from build123d import *

# Parameters (mm, degrees)
SKETCH1_R                = 1.6
SKETCH1_R_2              = 15.5
BOSS_EXTRUDE1_DEPTH      = 3
SKETCH2_W                = 12.85
SKETCH2_H                = 3
BOSS_EXTRUDE2_DEPTH      = 25
SKETCH3_R                = 1.6
CUT_EXTRUDE1_DEPTH       = 4
BOSS_EXTRUDE3_DEPTH      = 3
CHAMFER1_SIZE            = 2
FILLET1_R                = 3
FILLET2_R                = 3
CHAMFER1_OF_MIRROR1_SIZE = 2
FILLET1_OF_MIRROR1_R     = 3


with BuildPart() as part:
    # Sketch1 → Boss-Extrude1 (new body)
    with BuildSketch(Plane(origin=(0, 0, 0), x_dir=(1, 0, 0), z_dir=(0, 1, 0))):
        Polygon((46.15, 13.849265428), (-46.15, 13.849265428), (-59, -25.450734572), (-59, -28.450734572), (59, -28.450734572), (59, -25.450734572), align=None)
        with Locations((-40.5, 8.199265428)):
            Circle(SKETCH1_R, mode=Mode.SUBTRACT)
        with Locations((-9.5, 8.199265428)):
            Circle(SKETCH1_R, mode=Mode.SUBTRACT)
        with Locations((-40.5, -22.800734572)):
            Circle(SKETCH1_R, mode=Mode.SUBTRACT)
        with Locations((-9.5, -22.800734572)):
            Circle(SKETCH1_R, mode=Mode.SUBTRACT)
        with Locations((-25, -7.300734572)):
            Circle(SKETCH1_R_2, mode=Mode.SUBTRACT)
        with Locations((40.5, -22.800734572)):
            Circle(SKETCH1_R, mode=Mode.SUBTRACT)
        with Locations((9.5, -22.800734572)):
            Circle(SKETCH1_R, mode=Mode.SUBTRACT)
        with Locations((9.5, 8.199265428)):
            Circle(SKETCH1_R, mode=Mode.SUBTRACT)
        with Locations((40.5, 8.199265428)):
            Circle(SKETCH1_R, mode=Mode.SUBTRACT)
        with Locations((25, -7.300734572)):
            Circle(SKETCH1_R_2, mode=Mode.SUBTRACT)
    extrude(amount=BOSS_EXTRUDE1_DEPTH)

    # Sketch2 → Boss-Extrude2 (add)
    with BuildSketch(Plane(origin=(0, 3, 0), x_dir=(1, 0, 0), z_dir=(0, 1, 0))):
        with Locations((-52.575, -26.950734572)):
            Rectangle(SKETCH2_W, SKETCH2_H)
    boss_extrude2 = extrude(amount=BOSS_EXTRUDE2_DEPTH)

    # Sketch3 → Cut-Extrude1 (cut, through all)
    with BuildSketch(Plane(origin=(0, 0, 25.450734572), x_dir=(-1, 0, 0), z_dir=(0, 0, -1))):
        with Locations((55, 8)):
            Circle(SKETCH3_R)
        with Locations((55, 23)):
            Circle(SKETCH3_R)
    cut_extrude1 = extrude(amount=-CUT_EXTRUDE1_DEPTH, mode=Mode.SUBTRACT)

    # Sketch4 → Boss-Extrude3 (add)
    with BuildSketch(Plane(origin=(-46.15, 0, 0), x_dir=(0, 0, -1), z_dir=(1, 0, 0))):
        Polygon((-25.450734572, 28), (-0.450734572, 3), (-25.450734572, 3), align=None)
    boss_extrude3 = extrude(amount=-BOSS_EXTRUDE3_DEPTH)

    # Chamfer1
    chamfer1_edges = [part.edges().sort_by_distance(p)[0] for p in [
        (-49.15, 15.5, 25.450734572),
    ]]
    chamfer(chamfer1_edges, length=CHAMFER1_SIZE)

    # Fillet1
    fillet1_edges = [part.edges().sort_by_distance(p)[0] for p in [
        (-59, 28, 26.950734572),
    ]]
    fillet(fillet1_edges, radius=FILLET1_R)

    # Fillet2
    fillet2_edges = [part.edges().sort_by_distance(p)[0] for p in [
        (-46.15, 1.5, -13.849265428),
        (46.15, 1.5, -13.849265428),
    ]]
    fillet(fillet2_edges, radius=FILLET2_R)

    # Mirror1: Boss-Extrude2, Cut-Extrude1, Boss-Extrude3 across plane
    add(boss_extrude2.mirror(Plane(origin=(0, 0, 0), x_dir=(0, 0, 1), z_dir=(1, 0, 0))))
    add(cut_extrude1.mirror(Plane(origin=(0, 0, 0), x_dir=(0, 0, 1), z_dir=(1, 0, 0))), mode=Mode.SUBTRACT)
    add(boss_extrude3.mirror(Plane(origin=(0, 0, 0), x_dir=(0, 0, 1), z_dir=(1, 0, 0))))

    # Chamfer1 of Mirror1
    chamfer1_of_mirror1_edges = [part.edges().sort_by_distance(p)[0] for p in [
        (49.15, 15.5, 25.450734572),
    ]]
    chamfer(chamfer1_of_mirror1_edges, length=CHAMFER1_OF_MIRROR1_SIZE)

    # Fillet1 of Mirror1
    fillet1_of_mirror1_edges = [part.edges().sort_by_distance(p)[0] for p in [
        (59, 28, 26.950734572),
    ]]
    fillet(fillet1_of_mirror1_edges, radius=FILLET1_OF_MIRROR1_R)


solid = part.part
Geometry: final body of the model. Coordinates: model frame, mm. A direction names the side the tool comes from. Round coordinates to 2 decimals unless told otherwise and drop trailing zeros. Order: outer loops, then holes, each group sorted by start corner. A loop starts at its lowest first (then second) coordinate and runs counter-clockwise, first axis right, second up.
Q1. Section B-B, the plane y = 18.5. Output: boundary loops of the cut face in (x, z).
Result sheet:
outline: (-59, 25.45) - (-51.15, 25.45) - (-49.15, 23.45) - (-49.15, 15.95) - (-46.15, 15.95) - (-46.15, 28.45) - (-59, 28.45) - close; (46.15, 15.95) - (49.15, 15.95) - (49.15, 23.45) - (51.15, 25.45) - (59, 25.45) - (59, 28.45) - (46.15, 28.45) - close
Q2. Mould query, pull axis Y, two halves, no side actions, for faces 1 (the face through (56.48, 7.39, 26.93)), 2 (the face through (-56.48, 7.39, 26.93)), 3 (the face through (-1, 0, 12)), 4 (the face through (45.714, 1.521, -13.293)). Classes: released by +Y, released by -Y, zero draft, split by the parting line, or undercut.
Result sheet:
face 1: undercut
face 2: undercut
face 3: released by -Y
face 4: zero draft
Q3. Pin query (flat end, axial travel): pin 1 (3.5 mm diameter, centred on x = 9.5, z = 22.8, fed in from +Y); pin 2 (6.5 mm diameter, centred on x = 54.5, y = 16, fed in from -Z); pin 3 (5 mm diameter, centred on x = -40.5, z = -8.2, fed in from -Y); pin 4 (18.5 mm diameter, centred on x = 25, z = 7.3, fed in from -Y). Return the tip coordinate at first contact, or that it passes through.
Result sheet:
pin 1: stops at y = 3
pin 2: stops at z = 25.45
pin 3: stops at y = 0
pin 4: passes through
Q4. Section D-D, the plane y = 8. Output: boundary loops of the cut face in (x, z), and give its area (3 significant figures).
Result sheet:
outline: (-59, 25.45) - (-56.6, 25.45) - (-56.6, 28.45) - (-59, 28.45) - close; (-53.4, 25.45) - (-51.15, 25.45) - (-49.15, 23.45) - (-49.15, 5.45) - (-46.15, 5.45) - (-46.15, 28.45) - (-53.4, 28.45) - close; (46.15, 5.45) - (49.15, 5.45) - (49.15, 23.45) - (51.15, 25.45) - (53.4, 25.45) - (53.4, 28.45) - (46.15, 28.45) - close; (56.6, 25.45) - (59, 25.45) - (59, 28.45) - (56.6, 28.45) - close
area: 182 mm2
Q5. Section A-A, the plane x = 25. Output: boundary loops of the cut face in (y, z).
Result sheet:
outline: (0, -13.85) - (3, -13.85) - (3, -8.2) - (0, -8.2) - close; (0, 22.8) - (3, 22.8) - (3, 28.45) - (0, 28.45) - close
Q6. Section C-C, the plane z = 1.5. Output: boundary loops of the cut face in (x, y), and give its area (3 significant figures).
Result sheet:
outline: (-51.17, 0) - (-39.37, 0) - (-39.37, 3) - (-46.15, 3) - (-46.15, 4.05) - (-49.15, 4.05) - (-49.15, 3) - (-51.17, 3) - close; (-10.63, 0) - (10.63, 0) - (10.63, 3) - (-10.63, 3) - close; (39.37, 0) - (51.17, 0) - (51.17, 3) - (49.15, 3) - (49.15, 4.05) - (46.15, 4.05) - (46.15, 3) - (39.37, 3) - close
area: 141 mm2
Q7. Access query for faces 5 (the face through (-50.2, 15.3, 24.5)), 6 (the face through (50.2, 15.3, 24.5)), 7 (the face through (-1, 3, 7)). Directions: +Z, -Z, +X, -X, +Y, -Y. A direction counts if a zero-diameter tool reaches every point of the face in a straight line with its end or side. Return the directions, or none.
Result sheet:
face 5: -Z, -X, +Y
face 6: -Z, +X, +Y
face 7: -Z, +Y
Q8. Material intervals for probe 1 along Y at (x, z) = (55, 26.65); probe 2 along X at (y, z) = (16.25, 20.5); probe 3 along X at (y, z) = (1.75, 16.5), sorted ascending.
Result sheet:
probe 1: y = 0 to 6.4, 9.6 to 21.4, 24.6 to 28
probe 2: x = -49.15 to -46.15, 46.15 to 49.15
probe 3: x = -56.07 to -37.47, -12.53 to 12.53, 37.47 to 56.07
